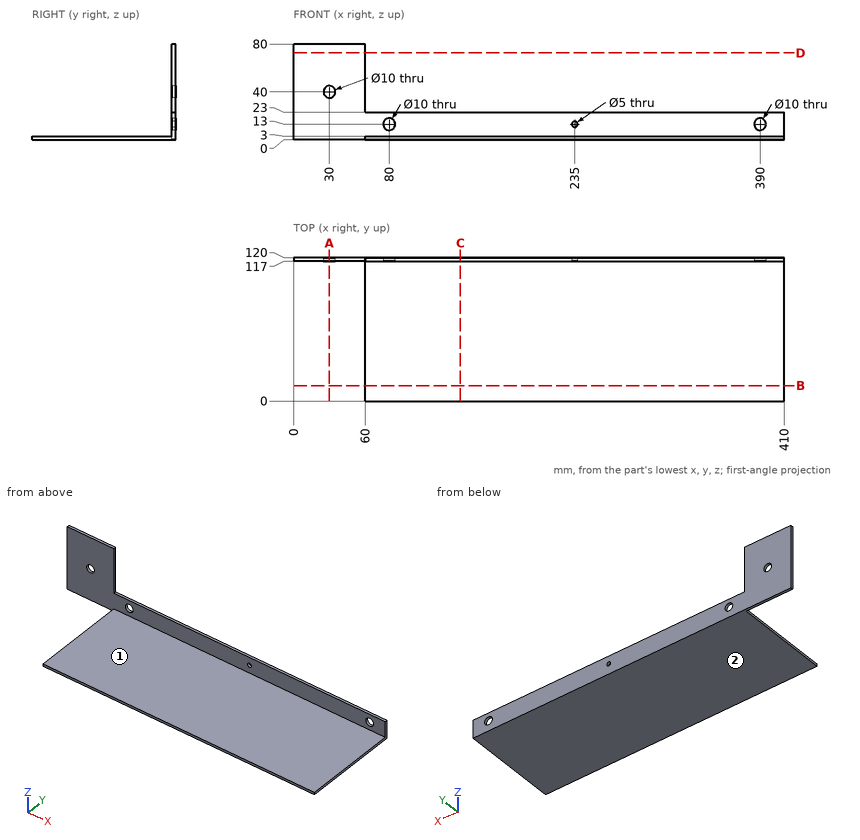
Here's the drawing with two shaded views (mm, measured from the low corner). I have some questions. A direction names the side the tool comes from. Give positions to 0.01 mm unless a question says otherwise; leave off trailing zeros. Write each loop counter-clockwise with the first axis right and the second up, starting at its lowest first coordinate (ties: lowest second). Pieces come first, ordered by that corner, then holes. Notation, with made-up numbers: (29, -6.75) -> (49, -6.75) arc R17 cw to (49, 9.25) -> close; hole circle Ø9 at (-3.5, 87.5). An arc over 180 degrees is marked (long way). One line per item, written item: value.
Q1. Which directions (+Z, -Z, +X, -X, +Y, -Y) give clear straight access to the entire face, cutting with the end or side of a thin tool? Please do the marked faces 1 and 2.
Results found:
face 1: +Z, +X, -X, -Y
face 2: -Z, +X, -X, +Y, -Y
Q2. Imagine slicing it at B-B on y = 13. Please give me the cut outline in (x, z), and give its area (3 significant figures).
Results found:
outline: (60, 0) -> (410, 0) -> (410, 3) -> (60, 3) -> close
area: 1,050 mm^2
Q3. For P1, Ø3.5, axis at y = 34, z = 1, coming from the -X side; P2, Ø8, axis at x = 80, z = 13, coming from the -Y side; P3, Ø8, axis at x = 202.5, y = 80.5, coming from the +Z side; P4, Ø2.5, axis at x = 273.5, y = 118, coming from the +Z side, each with a flat end and sliding along its axis, tell me the tip position at first contact or that it passes through.
Results found:
P1: stops at x = 60
P2: passes through
P3: stops at z = 3
P4: stops at z = 23
Q4. Imagine slicing it at D-D on z = 72.5. Please give me the cut outline in (x, y), and give its area (3 significant figures).
Results found:
outline: (0, 117) -> (60, 117) -> (60, 120) -> (0, 120) -> close
area: 180 mm^2
Q5. Imagine slicing it at C-C on x = 139.5. Please give me the cut outline in (y, z).
Results found:
outline: (0, 0) -> (120, 0) -> (120, 23) -> (117, 23) -> (117, 3) -> (0, 3) -> close
Q6. Imagine slicing it at A-A on x = 30. Please give me the cut outline in (y, z).
Results found:
outline: (117, 0) -> (120, 0) -> (120, 35) -> (117, 35) -> close; (117, 45) -> (120, 45) -> (120, 80) -> (117, 80) -> close
Q7. Please list where these lines run through material, in increasing order: line 1 (Z direction, x = 80, y = 118.15); line 2 (Z direction, x = 30, y = 118.4); line 3 (Z direction, x = 94.5, y = 5). Write a range as [from, to].
Results found:
line 1: z = [0, 8], [18, 23]
line 2: z = [0, 35], [45, 80]
line 3: z = [0, 3]
